Could you check a few things on this model? Use its own coordinates, in mm. Face numbers are marked on the shaded views. A direction names the side the tool comes from. Round coordinates to 2 decimals unless told otherwise and drop trailing zeros. Loops run counter-clockwise (first coordinate to the right, second up) from the corner with the lowest first, then second, coordinate; pieces in that order, holes last. Notation, with made-up numbers: (-15.5, 40) -> (-6.5, 40) arc R31 ccw to (-6.5, 73) -> close; hole circle Ø2 at (-29, -9.5). An arc over 180 degrees is marked (long way). Write each question's results on one line, items separated by ' | '. Start each with the question number.
1) Imagine slicing it at D-D, the plane y = -2.25. List the corners of the cut face in (x, z) for me.
2) Imagine slicing it at A-A, the plane z = 0. List the corners of the cut face in (x, y) for me.
3) For P1, Ø1, axis at y = -0.5, z = 13, coming from the +X side; P2, Ø2.5, axis at x = 0.5, z = -15, coming from the -Y side; P3, Ø1, axis at y = -0.5, z = 12, coming from the -X side, each with a flat end and sliding along its axis, tell me the tip position at first contact or that it passes through.
4) Which directions (+Z, -Z, +X, -X, +Y, -Y) give clear straight access to the entire face, cutting with the end or side of a thin tool? Please do the marked faces 1 and 2.
5) Imagine slicing it at C-C, the plane z = -12. List the corners of the cut face in (x, y) for me (3 decimals).
6) Imagine slicing it at B-B, the plane x = 0. List the corners of the cut face in (y, z) for me (3 decimals).
7) We'd pull the mould along X, two halves only. Please class the marked faces 3, 4, 5 and 6: pulls with the +X half, pulls with the -X half, needs draft (parallel to the pull), parting line crosses it, or undercut.
8) If I drill on probe 1 along Z at (x, y) = (1.5, 0); probe 2 along Y at (x, z) = (0, 12); probe 3 along Y at (x, z) = (0.75, 0), over which ranges is the centre line in solid material (lowest first)?
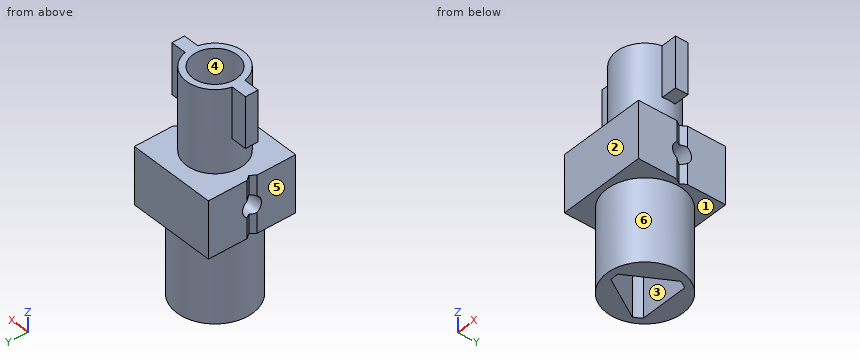
from build123d import *

# Parameters (mm, degrees)
F0_W      = 13.8
F0_H      = 13.8
F1_DEPTH  = 4.5
F2_R      = 4.5
F2_R_2    = 3.5
F3_DEPTH  = 13
F4_R      = 6
F5_DEPTH  = 13
F6_R      = 1.5
F7_DEPTH  = 13.801
F9_DEPTH  = 22.001
F10_W     = 3.2331479252
F10_H     = 2
F11_DEPTH = 8
F13_DEPTH = 9


with BuildPart() as f1:
    # F0 (on Top) → F1 (new body, symmetric)
    with BuildSketch(Plane.XY):
        Rectangle(F0_W, F0_H)
    extrude(amount=F1_DEPTH, both=True)

    # F2 (on face) → F3 (join)
    with BuildSketch(Plane.XY.offset(4.5)):
        Circle(F2_R)
        Circle(F2_R_2, mode=Mode.SUBTRACT)
    extrude(amount=F3_DEPTH)

    # F4 (on face) → F5 (join)
    with BuildSketch(Plane(origin=(0, 0, -4.5), x_dir=(1, 0, 0), z_dir=(0, 0, -1))):
        Circle(F4_R)
    extrude(amount=F5_DEPTH)

    # F6 (on face) → F7 (cut, through all)
    with BuildSketch(Plane.YZ.offset(6.9)):
        Circle(F6_R)
    extrude(amount=-F7_DEPTH, mode=Mode.SUBTRACT)

    # F8 (on face) → F9 (cut, through all)
    with BuildSketch(Plane(origin=(0, 0, -4.5), x_dir=(1, 0, 0), z_dir=(0, 0, -1))):
        Polygon((6.9, 0.8288529099), (6.3405334204, 0), (6.9, -0.8288529099), align=None)
        Polygon((-6.9, -0.7952927344), (-6.2937744095, 0), (-6.9, 0.7952927344), align=None)
    extrude(amount=-F9_DEPTH, mode=Mode.SUBTRACT)

    # F10 (on face) → F11 (join)
    with BuildSketch(Plane.XY.offset(17.5)):
        with Locations((-5.2334260374, 0)):
            Rectangle(F10_W, F10_H)
        with Locations((5.2334260374, 0)):
            Rectangle(F10_W, F10_H)
    extrude(amount=-F11_DEPTH)

    # F12 (on face) → F13 (cut)
    with BuildSketch(Plane(origin=(0, 0, -17.5), x_dir=(1, 0, 0), z_dir=(0, 0, -1))):
        with BuildLine():
            Line((4.51937948, -1.827794878), (0.6767729427, 4.827794878))
            ThreePointArc((0.6767729427, 4.827794878), (0, 4.875), (-0.6767729427, 4.827794878))
            Line((-0.6767729427, 4.827794878), (-4.51937948, -1.827794878))
            ThreePointArc((-4.51937948, -1.827794878), (-4.2218738434, -2.4375), (-3.8426065372, -3))
            Line((-3.8426065372, -3), (3.8426065372, -3))
            ThreePointArc((3.8426065372, -3), (4.2218738434, -2.4375), (4.51937948, -1.827794878))
        make_face()
    extrude(amount=-F13_DEPTH, mode=Mode.SUBTRACT)


solid = f1.part
Checked values:
1) outline: (-6.9, -4.5) -> (-5.56, -4.5) -> (-5.56, -17.5) -> (-2.17, -17.5) -> (-2.17, -8.5) -> (2.17, -8.5) -> (2.17, -17.5) -> (5.56, -17.5) -> (5.56, -4.5) -> (6.9, -4.5) -> (6.9, 4.5) -> (3.9, 4.5) -> (3.9, 17.5) -> (2.68, 17.5) -> (2.68, 4.5) -> (-2.68, 4.5) -> (-2.68, 17.5) -> (-3.9, 17.5) -> (-3.9, 4.5) -> (-6.9, 4.5) -> close
2) outline: (-6.9, -6.9) -> (6.9, -6.9) -> (6.9, -1.5) -> (-6.9, -1.5) -> close; (-6.9, 1.5) -> (6.9, 1.5) -> (6.9, 6.9) -> (-6.9, 6.9) -> close
3) P1: x = 6.85 | P2: y = -6 | P3: x = -6.85
4) face 1: -Z | face 2: +Z, -Z, +X, -X, -Y
5) outline: circle Ø12 at (0, 0); hole (-4.519, 1.828) -> (-0.677, -4.828) arc R4.875 ccw to (0.677, -4.828) -> (4.519, 1.828) arc R4.875 ccw to (3.843, 3) -> (-3.843, 3) arc R4.875 ccw to start
6) outline: (-6.9, -4.5) -> (-6, -4.5) -> (-6, -17.5) -> (-4.875, -17.5) -> (-4.875, -8.5) -> (3, -8.5) -> (3, -17.5) -> (6, -17.5) -> (6, -4.5) -> (6.9, -4.5) -> (6.9, 4.5) -> (4.5, 4.5) -> (4.5, 17.5) -> (3.5, 17.5) -> (3.5, 4.5) -> (-3.5, 4.5) -> (-3.5, 17.5) -> (-4.5, 17.5) -> (-4.5, 4.5) -> (-6.9, 4.5) -> close; hole circle Ø3 at (0, 0)
7) face 3: undercut | face 4: undercut | face 5: pulls with the -X half | face 6: parting line crosses it
8) probe 1: -8.5 to -1.5, 1.5 to 4.5 | probe 2: -4.5 to -3.5, 3.5 to 4.5 | probe 3: -6.9 to -1.5, 1.5 to 6.9
